```python
from build123d import *

# Parameters (mm, degrees)
F0_R     = 20
F1_DEPTH = 15
F2_R     = 18
F3_DEPTH = 13
F4_R     = 3.5
F4_R_2   = 1.5
F5_DEPTH = 15
F6_R     = 5
F7_DEPTH = 2


with BuildPart() as f1:
    # F0 (on Top) → F1 (new body)
    with BuildSketch(Plane.XY):
        Circle(F0_R)
    extrude(amount=F1_DEPTH)

    # F2 (on face) → F3 (cut)
    with BuildSketch(Plane.XY.offset(15)):
        Circle(F2_R)
    extrude(amount=-F3_DEPTH, mode=Mode.SUBTRACT)

    # F4 (on face) → F5 (join)
    with BuildSketch(Plane.XY.offset(2)):
        Circle(F4_R)
        Circle(F4_R_2, mode=Mode.SUBTRACT)
    extrude(amount=F5_DEPTH)

    # F6 (on face) → F7 (cut)
    with BuildSketch(Plane(origin=(0, 0, 0), x_dir=(1, 0, 0), z_dir=(0, 0, -1))):
        with Locations((10.725294, 0)):
            Circle(F6_R)
        with Locations((3.314298, -10.200361)):
            Circle(F6_R)
        with Locations((-8.676945, -6.30417)):
            Circle(F6_R)
        with Locations((-8.676945, 6.30417)):
            Circle(F6_R)
        with Locations((3.314298, 10.200361)):
            Circle(F6_R)
    extrude(amount=-F7_DEPTH, mode=Mode.SUBTRACT)


solid = f1.part
```
Input: part model. Units: mm. Frame: model coordinates. A direction names the side the tool comes from. Round coordinates to 2 decimals unless told otherwise and drop trailing zeros. Loops run counter-clockwise (first coordinate to the right, second up) from the corner with the lowest first, then second, coordinate; pieces in that order, holes last. Notation, with made-up numbers: (80.25, 59.5) -> (87.25, 59.5) arc R18 cw to (87.25, 75.5) -> close; hole circle Ø10 at (4, 0.25). An arc over 180 degrees is marked (long way). Use one line per item in the form item = value. Start each with the question number.
Item 1: Set-up query: faces 1 (the face through (3.233, -1.341, 9.395)), 2 (the face through (0, -2, 17)). Return all of +Z, -Z, +X, -X, +Y, -Y with unobstructed straight access to the full face (end or side cutting, diameter ignored); none if empty.
Item 2: Section query D-D on y = -8. Return the cut outline in (x, z).
Item 3: Section query C-C on x = 9. Return the cut outline in (y, z).
Item 4: Contact query for flat-ended pins moving along their axis: pin 1 Ø1.5 at (x, y) = (10.5, -11.5) entering from +Z; pin 2 Ø8 at (x, z) = (-10.5, 15) entering from +Y; pin 3 Ø8 at (x, y) = (-16, -12) entering from +Z; pin 4 Ø6 at (x, y) = (10.73, 0) entering from -Z. Output: stop coordinate, or through.
Item 5: Section query A-A on y = 0. Return the cut outline in (x, z), then the cut area to 3 significant figures.
Item 6: Mould query, pull axis Y, two halves, no side actions, for faces 3 (the face through (0, 0, 2)), 4 (the face through (0, 0, 0)), 5 (the face through (-4.336, -19.524, 7.395)). Classes: pulls with the +Y half, pulls with the -Y half, needs draft (parallel to the pull), parting line crosses it, or undercut.
Item 7: Section query B-B on z = 4. Return the cut outline in (x, y).
Item 8: Material intervals for L1, parallel to Z at x = -4.5, y = -2.5; L2, parallel to X at y = 0.5, z = 15.5; L3, parallel to X at y = -7, z = 7.75 (3 decimals), sorted ascending. Write a range as from..to.
Ans:
q1.face_1 = +Z
q1.face_2 = +Z, +X, -X, +Y, -Y
q2.outline = (-18.33, 0) -> (-13.38, 0) -> (-13.38, 2) -> (-16.12, 2) -> (-16.12, 15) -> (-18.33, 15) -> close; (-3.97, 0) -> (-1.18, 0) -> (-1.18, 2) -> (-3.97, 2) -> close; (7.8, 0) -> (18.33, 0) -> (18.33, 15) -> (16.12, 15) -> (16.12, 2) -> (7.8, 2) -> close
q3.outline = (-17.86, 0) -> (-4.69, 0) -> (-4.69, 2) -> (-15.59, 2) -> (-15.59, 15) -> (-17.86, 15) -> close; (4.69, 0) -> (17.86, 0) -> (17.86, 15) -> (15.59, 15) -> (15.59, 2) -> (4.69, 2) -> close
q4.pin_1 = 2
q4.pin_2 = 18.91
q4.pin_3 = 15
q4.pin_4 = through
q5.outline = (-20, 0) -> (5.73, 0) -> (5.73, 2) -> (3.5, 2) -> (3.5, 17) -> (1.5, 17) -> (1.5, 2) -> (-1.5, 2) -> (-1.5, 17) -> (-3.5, 17) -> (-3.5, 2) -> (-18, 2) -> (-18, 15) -> (-20, 15) -> close; (15.73, 0) -> (20, 0) -> (20, 15) -> (18, 15) -> (18, 2) -> (15.73, 2) -> close
q5.area = 172 mm^2
q6.face_3 = undercut
q6.face_4 = needs draft
q6.face_5 = parting line crosses it
q7.outline = circle Ø40 at (0, 0); circle Ø7 at (0, 0); hole circle Ø36 at (0, 0); hole circle Ø3 at (0, 0)
q8.L1 = 0..2
q8.L2 = -3.46..-1.41, 1.41..3.46
q8.L3 = -18.735..-16.583, 16.583..18.735
